Here's how the part is built. I have some questions about the finished solid (model axes, mm). A direction names the side the tool comes from. Give positions to 0.01 mm unless a question says otherwise; leave off trailing zeros. Write each loop counter-clockwise with the first axis right and the second up, starting at its lowest first coordinate (ties: lowest second). Pieces come first, ordered by that corner, then holes. Notation, with made-up numbers: M 5,44 L 21,44 A24 cw 21,58 Z; hole C 1,-25 d11. An arc over 180 degrees is marked long. Use one line per item in the form item = value. Start each with the question number.
Autodesk Inventor part; units mm, degrees
ref_plane "Work Plane2" through (8.89, 0, 0) normal (1, 0, 0) x (0, 0, -1)
ref_plane "Work Plane1" through (-12.7, 0, 0) normal (1, 0, 0) x (0, 0, -1)
ref_plane "YZ Plane" through (0, 0, 0) normal (1, 0, 0) x (0, 1, 0)
sketch "Sketch1" plane through (0, 0, 0) normal (1, 0, 0) x (0, 1, 0)
  circle A0 centre (0, 0) radius 19.05
  dimension "d0" = 38.1
extrude "Extrusion1" add sketch "Sketch1" along normal blind 12.7
sketch "Sketch10" plane through (12.7, 0, 0) normal (1, 0, 0) x (0, 0, -1)
  point P0 (0, 0)
  point P1 (0, 0)
hole "Hole4" at (12.7, 0, 0) direction (-1, 0, 0) diameter 10.3188 depth 3.81
ref_plane "Work Plane2" through (8.89, 0, 0) normal (1, 0, 0) x (0, 0, -1)
hole "Hole1" at (8.89, 0, 0) direction (-1, 0, 0) diameter 6.7469 depth 4.7625
ref_plane "Work Plane1" through (-12.7, 0, 0) normal (1, 0, 0) x (0, 0, -1)
sketch "Sketch5" plane through (0, 0, 0) normal (1, 0, 0) x (0, 1, 0)
  line L0 (0, 9) -> (0, -9)
  circle A0 centre (0, 0) radius 19.05
  line L1 (-9.525, 0) -> (9.525, 0)
  line L2 (-9.525, 7.62) -> (-9.525, -7.62)
  dimension "d37" = 18
  dimension "d45" = 19.05
  dimension "d46" = 15.24
hole "Hole2" at (0, 0, -9) direction (1, 0, 0) diameter 2.159 depth 8.8646 tip angle 118
sketch "Sketch6" plane through (0, 0, 0) normal (-1, 0, 0) x (0, 0, 1)
  circle A0 centre (0, 0) radius 0.5715
  dimension "d34" = 1.143
hole "Hole5" at (0, 0, 0) direction (1, 0, 0) diameter 1 end through all
mirror "Mirror1" about plane through (0, 0, 0) normal (0, 0, 1) of "Hole2"
hole "Hole3" at (0, -9.525, 7.62) at (0, -9.525, -7.62) direction (1, 0, 0) diameter 2.9464 end through all
mirror "Mirror2" about plane through (0, 0, 0) normal (0, 1, 0) of "Hole3"
sketch "Sketch9" plane through (0, 0, 0) normal (0, 1, 0) x (-1, 0, 0)
  line L0 (-11.4554, -6.2103) -> (-12.7, -6.2103)
  line L1 (-12.7, -6.2103) -> (-12.7, -8.7503)
  line L2 (-12.7, -8.7503) -> (-11.4554, -8.7503)
  line L3 (-11.4554, -8.7503) -> (-11.4554, -6.2103)
  line L4 (2.54, 0) -> (-15.24, 0)
  line L5 (-12.7, 19.05) -> (-12.7, -19.05)
  point P0 (0, 0)
  dimension "d55" = 2.54
  dimension "d56" = 1.2446
  dimension "d59" = 6.2103
revolve "Revolution1" cut sketch "Sketch9" angle 360 about axis through (-10, 0, 0) along (1, 0, 0)
properties part number "NuMu sensor" material "Aluminum 6061"
1) Suppose I cut it at A-A, the plane z = 0. List the corners of the cut face in (x, y) for me.
2) Suppose I cut it at B-B, the plane x = 5.75. State how many separate pieces and enclosed holes the cut face has, and give its area (3 significant figures).
3) Thinking about a two-plate mould opening in Z: for faces 4 (the face through (0, 4, 0)), 5 (the face through (6.44, 9.46, 6.15)), 6 (the face through (6.26, -15.12, 11.59)), which applies, released by +Z, released by -Z, zero draft, split by the parting line, or undercut?
4) On a 3-axis mill with a long thin cutter (end or side, diameter ignored), from which of +Z, -Z, +X, -X, +Y, -Y can I reach the whole of each face in a straight line? I mean faces 1 (the face through (4.49, 0.05, 10.08)), 2 (the face through (8.89, 1.1, -3.4)), 3 (the face through (6.4, 8.3, -6.8)). Say none if no direction works.
5) Suppose I cut it at C-C, the plane y = -4.5. List the corners of the cut face in (x, z) for me.
6) Will these pins go through, and if not, where does the flat tip stop? P1, Ø1, axis at x = 10.5, y = 9, coming from the -Z side; P2, Ø1.5, axis at x = 8.5, y = 4, coming from the +Z side; P3, Ø7.5, axis at y = -0.5, z = 0, coming from the +X side.
7) Please list where these lines run through material, in increasing order: line 1 (Z direction, x = 2.75, y = 0); line 2 (Z direction, x = 7.05, y = 0); line 3 (Y direction, x = 11.5, z = 2.5).
8) Suppose I cut it at D-D, the plane z = 14. List the corners of the cut face in (x, y) for me, and give its area (3 significant figures).
Checks:
q1.outline = M 0,-19.05 L 12.7,-19.05 L 12.7,-8.75 L 11.46,-8.75 L 11.46,-6.21 L 12.7,-6.21 L 12.7,-5.16 L 8.89,-5.16 L 8.89,-3.37 L 4.13,-3.37 L 4.13,-0.5 L 0,-0.5 Z; M 0,0.5 L 4.13,0.5 L 4.13,3.37 L 8.89,3.37 L 8.89,5.16 L 12.7,5.16 L 12.7,6.21 L 11.46,6.21 L 11.46,8.75 L 12.7,8.75 L 12.7,19.05 L 0,19.05 Z
q2.separate_pieces = 1
q2.enclosed_holes = 7
q2.area = 1,070 mm^2
q3.face_4 = zero draft
q3.face_5 = undercut
q3.face_6 = split by the parting line
q4.face_1 = -X
q4.face_2 = +X
q4.face_3 = +X, -X
q5.outline = M 0,-18.51 L 12.7,-18.51 L 12.7,-7.5 L 11.46,-7.5 L 11.46,-4.28 L 12.7,-4.28 L 12.7,-2.52 L 8.89,-2.52 L 8.89,2.52 L 12.7,2.52 L 12.7,4.28 L 11.46,4.28 L 11.46,7.5 L 12.7,7.5 L 12.7,18.51 L 0,18.51 Z
q6.P1 = -17.05
q6.P2 = 18.77
q6.P3 = 8.89
q7.line_1 = -19.05 to -10.08, -7.92 to -0.5, 0.5 to 7.92, 10.08 to 19.05
q7.line_2 = -19.05 to -10.08, -7.92 to -3.37, 3.37 to 7.92, 10.08 to 19.05
q7.line_3 = -18.89 to -8.39, -5.68 to -4.51, 4.51 to 5.68, 8.39 to 18.89
q8.outline = M 0,-12.92 L 12.7,-12.92 L 12.7,12.92 L 0,12.92 Z
q8.area = 328 mm^2
